from build123d import *

# Parameters (mm, degrees)
F3_W     = 34
F3_H     = 94
F4_DEPTH = 500
F6_D     = 12
F6_DEPTH = 40
F6_TIP   = 3.6051637142
F7_DEPTH = 40
F8_DEPTH = 35
F9_DEPTH = 35


# Not quite as in the source:
# - a feature names something its author has since deleted; it is built from what else it names


with BuildPart() as f4:
    # F3 (on Right) → F4 (new body, symmetric)
    with BuildSketch(Plane.YZ):
        with BuildLine():
            ThreePointArc((-4.2945303673, -84.5), (-3.7087439297, -85.9142135624), (-2.2945303673, -86.5))
            Line((-2.2945303673, -86.5), (33.7054696327, -86.5))
            ThreePointArc((33.7054696327, -86.5), (35.1196831951, -85.9142135624), (35.7054696327, -84.5))
            Line((35.7054696327, -84.5), (35.7054696327, 11.5))
            ThreePointArc((35.7054696327, 11.5), (35.1196831951, 12.9142135624), (33.7054696327, 13.5))
            Line((33.7054696327, 13.5), (-2.2945303673, 13.5))
            ThreePointArc((-2.2945303673, 13.5), (-3.7087439297, 12.9142135624), (-4.2945303673, 11.5))
            Line((-4.2945303673, 11.5), (-4.2945303673, -84.5))
        make_face()
        with Locations((15.7054696327, -36.5)):
            Rectangle(F3_W, F3_H, mode=Mode.SUBTRACT)
    extrude(amount=F4_DEPTH, both=True)

    # F6
    with Locations(Plane.XZ.offset(4.2945303673)):
        with Locations((450, -36.2195856869), (0, -36.2195856869), (-450, -36.5)):
            Hole(F6_D / 2, depth=F6_DEPTH)
            with Locations((0, 0, -(F6_DEPTH + F6_TIP / 2))):  # 118° drill point
                Cone(0, F6_D / 2, F6_TIP, mode=Mode.SUBTRACT)

    # F5 (on face) → F7 (cut)
    with BuildSketch(Plane.XZ.offset(4.2945303673)):
        with BuildLine():
            ThreePointArc((-500, -36.5), (-490, -6.5), (-464, 11.5))
            Line((-464, 11.5), (-500, 11.5))
            Line((-500, 11.5), (-500, -36.5))
        make_face()
        with BuildLine():
            ThreePointArc((-464, -84.5), (-490, -66.5), (-500, -36.5))
            Line((-500, -36.5), (-500, -84.5))
            Line((-500, -84.5), (-464, -84.5))
        make_face()
        with BuildLine():
            Line((500, 11.5), (464, 11.5))
            ThreePointArc((464, 11.5), (490, -6.5), (500, -36.5))
            Line((500, -36.5), (500, 11.5))
        make_face()
        with BuildLine():
            Line((500, -84.5), (500, -36.5))
            ThreePointArc((500, -36.5), (490, -66.5), (464, -84.5))
            Line((464, -84.5), (500, -84.5))
        make_face()
    extrude(amount=-F7_DEPTH, mode=Mode.SUBTRACT)

    # F8 (cut): faces of the model
    f8_faces = [f4.faces().sort_by_distance(p)[0] for p in [
        (-500, 15.7054696327, 12.4878664624),
        (-500, 15.7054696327, -85.4878664624),
    ]]
    extrude(f8_faces, amount=-F8_DEPTH, mode=Mode.SUBTRACT)

    # F9 (cut): faces of the model
    f9_faces = [f4.faces().sort_by_distance(p)[0] for p in [
        (500, 15.7054696327, -85.4878664624),
        (500, 15.7054696327, 12.4878664624),
    ]]
    extrude(f9_faces, amount=-F9_DEPTH, mode=Mode.SUBTRACT)


solid = f4.part
Input: part model. Units: mm. Frame: model coordinates. A direction names the side the tool comes from. Coordinates: 2 decimals unless noted, no trailing zeros. Loops run counter-clockwise (first coordinate to the right, second up) from the corner with the lowest first, then second, coordinate; pieces in that order, holes last. Notation, with made-up numbers: (-37, -21) -> (-29, -21) arc R25 ccw to (-29, -5) -> close; hole circle Ø9 at (73.5, 55.5). An arc over 180 degrees is marked (long way). Write each question's results on one line, items separated by ' | '. Start each with the question number.
Q1. Pin query (flat end, axial travel): pin 1 (7 mm diameter, centred on x = 450, z = -36.22, fed in from +Y); pin 2 (1 mm diameter, centred on y = 22, z = 12.5, fed in from -X); pin 3 (2 mm diameter, centred on y = 14, z = -86, fed in from +X). Return the tip coordinate at first contact, or that it passes through.
Q2. Section A-A, the plane y = 11. Return the cut outline in (x, z), plus the area to 3 significant figures.
Q3. Reachability of faces 4 (the flat face through (7, -4.295, -36)), 5 (the flat face through (7, 15, -83.5)) from +Z, -Z, +X, -X, +Y, -Y: full face, straight path, thin tool, end or side. Return the list, or none.
Q4. Pull-direction query (Z, two-part tool) for faces 1 (the flat face through (7, 32.705, -37)), 2 (the flat face through (7, 35.705, -37)), 3 (the flat face through (7, 15, -86.5)); classes: released by +Z, released by -Z, zero draft, split by the parting line, or undercut.
Q5. Section C-C, the plane x = -270.5. Return the cut outline in (y, z).
Q6. Ray query, line 1 (X direction, y = -2, z = -36); line 2 (Z direction, x = 373.5, y = 4.5); line 3 (Y direction, x = -188, z = -13.5). Return the intervals inside material, ascending. Write a range as from..to.
Q7. Section D-D, the plane z = -58. Return the cut outline in (x, y).
Q8. Section B-B, the plane z = -19. Return the cut outline in (x, y).
Found:
1) pin 1: through | pin 2: x = -465 | pin 3: x = 465
2) outline: (-467.06, -83.5) arc R50 ccw to (-464, -84.5) -> (-465, -84.5) -> (-465, -86.5) -> (465, -86.5) -> (465, -84.5) -> (464, -84.5) arc R50 ccw to (467.06, -83.5) -> close; (-467.06, 10.5) -> (467.06, 10.5) arc R50 ccw to (464, 11.5) -> (465, 11.5) -> (465, 13.5) -> (-465, 13.5) -> (-465, 11.5) -> (-464, 11.5) arc R50 ccw to start | area: 5,580 mm2
3) face 4: +Z, -Z, +X, -X, -Y | face 5: +X, -X
4) face 1: undercut | face 2: zero draft | face 3: released by -Z
5) outline: (-4.29, -84.5) arc R2 ccw to (-2.29, -86.5) -> (33.71, -86.5) arc R2 ccw to (35.71, -84.5) -> (35.71, 11.5) arc R2 ccw to (33.71, 13.5) -> (-2.29, 13.5) arc R2 ccw to (-4.29, 11.5) -> close; hole (-1.29, -83.5) -> (32.71, -83.5) -> (32.71, 10.5) -> (-1.29, 10.5) -> close
6) line 1: -500..-455.98, -444.02..-6, 6..444, 456..500 | line 2: -86.5..-83.5, 10.5..13.5 | line 3: -4.29..-1.29, 32.71..35.71
7) outline: (-495.14, -4.29) -> (495.14, -4.29) -> (495.14, -1.29) -> (-495.14, -1.29) -> close; (-495.14, 32.71) -> (495.14, 32.71) -> (495.14, 35.71) -> (-495.14, 35.71) -> close
8) outline: (-496.84, -4.29) -> (496.84, -4.29) -> (496.84, -1.29) -> (-496.84, -1.29) -> close; (-496.84, 32.71) -> (496.84, 32.71) -> (496.84, 35.71) -> (-496.84, 35.71) -> close
